Could you check a few things on this model? Use its own coordinates, in mm. Coordinates: 2 decimals unless noted, no trailing zeros. Order: outer loops, then holes, each group sorted by start corner. A loop starts at its lowest first (then second) coordinate and runs counter-clockwise, first axis right, second up. Notation, with made-up numbers: (43, -4.75) -> (84, -4.75) arc R23 ccw to (84, 24.25) -> close; hole circle Ø2 at (57.5, 16.25). An arc over 180 degrees is marked (long way). Put each result on its own line as item: value. Start each with the question number.
Q1. If we section it at B-B (z = 237.5): Please give me the cut outline in (x, y).
Q2. We'd pull the mould along Y, two halves only. Please class faces 1 (the face through (-152.26, -146.05, 6.06)), 2 (the face through (152.26, 146.05, 6.06)), 3 (the face through (174.626, 0.093, 4.712)), 4 (the face through (-174.626, -0.093, 4.042)): +Y half, -Y half, draft (parallel to the pull), parting line (faces both ways), or undercut.
Q3. Please list where these lines run through material, in increasing order: line 1 along Y through (x, z) = (46.5, 23); line 2 along Y through (x, z) = (-101, 123.5); line 3 along X through (y, z) = (-3.5, 14).
Q4. If we section it at D-D (z = 198): Please give me the cut outline in (x, y), and give its area (3 significant figures).
Q5. Will these pins go through, and if not, where does the flat tip stop? pin 1 (8 mm diameter, centred on x = -71, z = 80.5, fed in from +Y); pin 2 (1 mm diameter, centred on y = 95, z = 139.5, fed in from +X); pin 3 (12 mm diameter, centred on y = 109.5, z = 47.5, fed in from -X).
from build123d import *
from OCP.BRepFilletAPI import BRepFilletAPI_MakeChamfer

# Parameters (mm, degrees)
SKETCH1_W           = 355.6
SKETCH1_H           = 304.8
BOSS_EXTRUDE1_DEPTH = 254
CHAMFER1_SIZE       = 254
CHAMFER1_SIZE_2     = 101.6
CHAMFER2_SIZE       = 254
CHAMFER2_SIZE_2     = 76.2
SKETCH2_R           = 6.35
CUT_EXTRUDE1_DEPTH  = 346.477350922


with BuildPart() as part:
    # Sketch1 → Boss-Extrude1 (new body)
    with BuildSketch(Plane.XY):
        Rectangle(SKETCH1_W, SKETCH1_H)
    extrude(amount=BOSS_EXTRUDE1_DEPTH)

    # Chamfer1
    chamfer1_edges_1 = [part.edges().sort_by_distance(p)[0] for p in [
        (0, -152.4, 254),
    ]]
    chamfer1_side_1 = [part.faces().sort_by_distance(p)[0] for p in [
        (0, -152.4, 251.968),
    ]]
    chamfer1_edges_2 = [part.edges().sort_by_distance(p)[0] for p in [
        (0, 152.4, 254),
    ]]
    chamfer1_side_2 = [part.faces().sort_by_distance(p)[0] for p in [
        (0, 152.4, 251.968),
    ]]
    chamfer1 = BRepFilletAPI_MakeChamfer(part.part.solid().wrapped)
    for e in chamfer1_edges_1:
        chamfer1.Add(CHAMFER1_SIZE - 0.0001, CHAMFER1_SIZE_2 - 0.0001, e.wrapped, chamfer1_side_1[0].wrapped)
    for e in chamfer1_edges_2:
        chamfer1.Add(CHAMFER1_SIZE - 0.0001, CHAMFER1_SIZE_2 - 0.0001, e.wrapped, chamfer1_side_2[0].wrapped)
    add(Compound.cast(chamfer1.Shape()), mode=Mode.REPLACE)  # a hair under: the kernel refuses the full size

    # Chamfer2
    chamfer2_edges_1 = [part.edges().sort_by_distance(p)[0] for p in [
        (177.8, 0, 254),
    ]]
    chamfer2_side_1 = [part.faces().sort_by_distance(p)[0] for p in [
        (177.8, 0, 252.476),
    ]]
    chamfer2_edges_2 = [part.edges().sort_by_distance(p)[0] for p in [
        (-177.8, 0, 254),
    ]]
    chamfer2_side_2 = [part.faces().sort_by_distance(p)[0] for p in [
        (-177.8, 0, 252.476),
    ]]
    chamfer2 = BRepFilletAPI_MakeChamfer(part.part.solid().wrapped)
    for e in chamfer2_edges_1:
        chamfer2.Add(CHAMFER2_SIZE - 0.0001, CHAMFER2_SIZE_2 - 0.0001, e.wrapped, chamfer2_side_1[0].wrapped)
    for e in chamfer2_edges_2:
        chamfer2.Add(CHAMFER2_SIZE - 0.0001, CHAMFER2_SIZE_2 - 0.0001, e.wrapped, chamfer2_side_2[0].wrapped)
    add(Compound.cast(chamfer2.Shape()), mode=Mode.REPLACE)  # a hair under: the kernel refuses the full size

    # Sketch2 → Cut-Extrude1 (cut, through all)
    with BuildSketch(Plane.XY):
        with Locations((-180.975, 0)):
            Circle(SKETCH2_R)
        with Locations((0, 152.4)):
            Circle(SKETCH2_R)
        with Locations((152.4, 152.4)):
            Circle(SKETCH2_R)
        with Locations((-152.4, 152.4)):
            Circle(SKETCH2_R)
        with Locations((180.975, 0)):
            Circle(SKETCH2_R)
        with Locations((152.4, -152.4)):
            Circle(SKETCH2_R)
        with Locations((0, -152.4)):
            Circle(SKETCH2_R)
        with Locations((-152.4, -152.4)):
            Circle(SKETCH2_R)
    extrude(amount=CUT_EXTRUDE1_DEPTH, mode=Mode.SUBTRACT)


solid = part.part
The answers:
1. outline: (-106.55, -57.4) -> (106.55, -57.4) -> (106.55, 57.4) -> (-106.55, 57.4) -> close
2. face 1: -Y half
2. face 2: +Y half
2. face 3: undercut
2. face 4: undercut
3. line 1: -143.2 to 143.2
3. line 2: -103 to 103
3. line 3: -173.6 to 173.6
4. outline: (-118.4, -73.2) -> (118.4, -73.2) -> (118.4, 73.2) -> (-118.4, 73.2) -> close
4. area: 34,700 mm^2
5. pin 1: y = 121.8
5. pin 2: x = 136.1
5. pin 3: x = -165.35
